Check sheet for the modelled part. Datum: model origin and axes. Units: mm. Face numbers are marked on the shaded views. Round coordinates to 2 decimals unless told otherwise and drop trailing zeros. Write each loop counter-clockwise with the first axis right and the second up, starting at its lowest first coordinate (ties: lowest second). Pieces come first, ordered by that corner, then holes. Notation, with made-up numbers: (19, 24) -> (65, 24) arc R21 ccw to (65, 44) -> close; hole circle Ø6 at (54.5, -36). An arc over 180 degrees is marked (long way). Answer as a JSON object with one key per item and string values. Group by question number.
```python
from build123d import *

# Parameters (mm, degrees)
BOSS_EXTRUDE1_START  = -59.6
SKETCH1_R            = 9
BOSS_EXTRUDE1_DEPTH  = 4
BOSS_EXTRUDE2_START  = -58
SKETCH2_W            = 4
SKETCH2_H            = 49
BOSS_EXTRUDE2_DEPTH  = 12
BOSS_EXTRUDE3_START  = -76.9
SKETCH3_W            = 4
SKETCH3_H            = 22
BOSS_EXTRUDE3_DEPTH  = 39
BOSS_EXTRUDE4_START  = -57.4
SKETCH4_R            = 4.6
BOSS_EXTRUDE4_DEPTH  = 2.3
BOSS_EXTRUDE5_START  = -55.3
SKETCH5_W            = 2.3
SKETCH5_H            = 17.5
BOSS_EXTRUDE5_DEPTH  = 6.6
BOSS_EXTRUDE6_START  = -52.9
SKETCH6_W            = 6
SKETCH6_H            = 10.5
BOSS_EXTRUDE6_DEPTH  = 1.8
BOSS_EXTRUDE7_START  = -55.3
SKETCH7_W            = 2.3
SKETCH7_H            = 17.5
BOSS_EXTRUDE7_DEPTH  = 6.6
BOSS_EXTRUDE8_START  = -52.9
SKETCH8_W            = 6
SKETCH8_H            = 10.5
BOSS_EXTRUDE8_DEPTH  = 1.8
BOSS_EXTRUDE9_START  = -60.6
SKETCH9_R            = 3
BOSS_EXTRUDE9_DEPTH  = 6
BOSS_EXTRUDE10_START = -69.1
SKETCH10_W           = 6
SKETCH10_H           = 13
BOSS_EXTRUDE10_DEPTH = 23.4
BOSS_EXTRUDE11_START = -72.925
SKETCH11_W           = 6
SKETCH11_H           = 2
BOSS_EXTRUDE11_DEPTH = 2.9
BOSS_EXTRUDE12_START = -44.775
SKETCH12_W           = 6
SKETCH12_H           = 2
BOSS_EXTRUDE12_DEPTH = 2.9


with BuildPart() as part:
    # Sketch1 → Boss-Extrude1 (new body)
    with BuildSketch(Plane(origin=(0, 0, 0), x_dir=(0, 0, -1), z_dir=(1, 0, 0)).offset(BOSS_EXTRUDE1_START)):
        with Locations((52, 18)):
            Circle(SKETCH1_R)
    extrude(amount=BOSS_EXTRUDE1_DEPTH)

    # Sketch2 → Boss-Extrude2 (add)
    with BuildSketch(Plane.XY.offset(BOSS_EXTRUDE2_START)):
        with Locations((-57.6, 12.5)):
            Rectangle(SKETCH2_W, SKETCH2_H)
    extrude(amount=BOSS_EXTRUDE2_DEPTH)

    # Sketch3 → Boss-Extrude3 (add)
    with BuildSketch(Plane.XY.offset(BOSS_EXTRUDE3_START)):
        with Locations((-57.6, -20)):
            Rectangle(SKETCH3_W, SKETCH3_H)
    extrude(amount=BOSS_EXTRUDE3_DEPTH)


with BuildPart() as body_2:
    # Sketch4 → Boss-Extrude4 (new body)
    with BuildSketch(Plane(origin=(0, 0, 0), x_dir=(0, 0, -1), z_dir=(1, 0, 0)).offset(BOSS_EXTRUDE4_START)):
        with Locations((52, 18)):
            Circle(SKETCH4_R)
    extrude(amount=BOSS_EXTRUDE4_DEPTH)


with BuildPart() as part_1:
    add(part.part)

    # Combine1: cut body 2
    add(body_2.part, mode=Mode.SUBTRACT)


with BuildPart() as body_2_2:
    # Sketch5 → Boss-Extrude5 (new body)
    with BuildSketch(Plane.XY.offset(BOSS_EXTRUDE5_START)):
        with Locations((-56.25, 26.75)):
            Rectangle(SKETCH5_W, SKETCH5_H)
    extrude(amount=BOSS_EXTRUDE5_DEPTH)


with BuildPart() as part_2:
    add(part_1.part)

    # Combine2: cut body 2 2
    add(body_2_2.part, mode=Mode.SUBTRACT)


with BuildPart() as body_2_3:
    # Sketch6 → Boss-Extrude6 (new body)
    with BuildSketch(Plane.XY.offset(BOSS_EXTRUDE6_START)):
        with Locations((-57.6, 28.75)):
            Rectangle(SKETCH6_W, SKETCH6_H)
    extrude(amount=BOSS_EXTRUDE6_DEPTH)


with BuildPart() as part_3:
    add(part_2.part)

    # Combine3: cut body 2 3
    add(body_2_3.part, mode=Mode.SUBTRACT)


with BuildPart() as body_2_4:
    # Sketch7 → Boss-Extrude7 (new body)
    with BuildSketch(Plane.XY.offset(BOSS_EXTRUDE7_START)):
        with Locations((-56.25, 9.25)):
            Rectangle(SKETCH7_W, SKETCH7_H)
    extrude(amount=BOSS_EXTRUDE7_DEPTH)


with BuildPart() as part_4:
    add(part_3.part)

    # Combine4: cut body 2 4
    add(body_2_4.part, mode=Mode.SUBTRACT)


with BuildPart() as body_2_5:
    # Sketch8 → Boss-Extrude8 (new body)
    with BuildSketch(Plane.XY.offset(BOSS_EXTRUDE8_START)):
        with Locations((-57.6, 7.25)):
            Rectangle(SKETCH8_W, SKETCH8_H)
    extrude(amount=BOSS_EXTRUDE8_DEPTH)


with BuildPart() as part_5:
    add(part_4.part)

    # Combine5: cut body 2 5
    add(body_2_5.part, mode=Mode.SUBTRACT)


with BuildPart() as body_2_6:
    # Sketch9 → Boss-Extrude9 (new body)
    with BuildSketch(Plane(origin=(0, 0, 0), x_dir=(0, 0, -1), z_dir=(1, 0, 0)).offset(BOSS_EXTRUDE9_START)):
        with Locations((52, 18)):
            Circle(SKETCH9_R)
    extrude(amount=BOSS_EXTRUDE9_DEPTH)


with BuildPart() as part_6:
    add(part_5.part)

    # Combine6: cut body 2 6
    add(body_2_6.part, mode=Mode.SUBTRACT)


with BuildPart() as body_2_7:
    # Sketch10 → Boss-Extrude10 (new body)
    with BuildSketch(Plane.XY.offset(BOSS_EXTRUDE10_START)):
        with Locations((-57.6, -20)):
            Rectangle(SKETCH10_W, SKETCH10_H)
    extrude(amount=BOSS_EXTRUDE10_DEPTH)


with BuildPart() as part_7:
    add(part_6.part)

    # Combine7: cut body 2 7
    add(body_2_7.part, mode=Mode.SUBTRACT)


with BuildPart() as body_2_8:
    # Sketch11 → Boss-Extrude11 (new body)
    with BuildSketch(Plane.XY.offset(BOSS_EXTRUDE11_START)):
        with Locations((-57.6, -20)):
            Rectangle(SKETCH11_W, SKETCH11_H)
    extrude(amount=BOSS_EXTRUDE11_DEPTH)


with BuildPart() as part_8:
    add(part_7.part)

    # Combine8: cut body 2 8
    add(body_2_8.part, mode=Mode.SUBTRACT)


with BuildPart() as body_2_9:
    # Sketch12 → Boss-Extrude12 (new body)
    with BuildSketch(Plane.XY.offset(BOSS_EXTRUDE12_START)):
        with Locations((-57.6, -20)):
            Rectangle(SKETCH12_W, SKETCH12_H)
    extrude(amount=BOSS_EXTRUDE12_DEPTH)


with BuildPart() as part_9:
    add(part_8.part)

    # Combine9: cut body 2 9
    add(body_2_9.part, mode=Mode.SUBTRACT)


solid = part_9.part
```
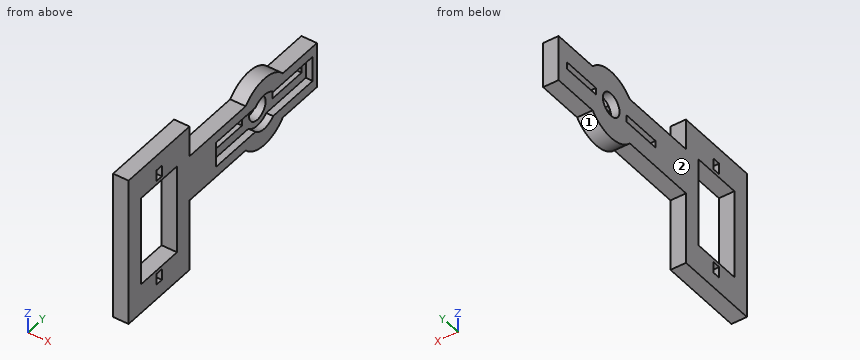
(1) Release check for a two-part mould opening along Y. For the marked faces 1 and 2 record: pulls with the +Y half, pulls with the -Y half, needs draft (parallel to the pull), parting line crosses it, or undercut.
(2) Section check A-A on x = -56.5. State how many separate pieces and enclosed holes the cut face has, then the cut area to 3 significant figures.
(3) Section check C-C on y = 8.5. Record the cut outline in (x, z), then the cut area to 3 significant figures.
(4) Scan lines: line 1 along Y through (x, z) = (-58.6, -52); line 2 along Z through (x, y) = (-57.7, 9.5); line 3 along Y through (x, z) = (-58.2, -68). Record each from-to range of solid material in increasing order.
(5) Section check B-B on z = -52. Record the cut outline in (x, y).
(6) Section check D-D on y = 18. Record the cut outline in (x, z).
(7) Go/stop test with flat-tipped pins: pin 1 Ø0.9 at (x, y) = (-56.5, 28.5) entering from -Z; pin 2 Ø0.9 at (x, y) = (-56.5, 4.5) entering from +Z; pin 3 Ø1.5 at (x, z) = (-56.5, -71.5) entering from +Y. Record where each tip stops, or that it passes through.
Data:
{
 "1": {"face 1": "undercut", "face 2": "needs draft"},
 "2": {"separate pieces": "1", "enclosed holes": "4", "area": "907 mm²"},
 "3": {"outline": "(-59.6, -58) -> (-55.6, -58) -> (-55.6, -55.3) -> (-57.4, -55.3) -> (-57.4, -52.9) -> (-59.6, -52.9) -> close; (-59.6, -51.1) -> (-57.4, -51.1) -> (-57.4, -48.7) -> (-55.6, -48.7) -> (-55.6, -46) -> (-59.6, -46) -> close", "area": "32.2 mm²"},
 "4": {"line 1": "y = -31 to -26.5, -13.5 to 2, 12.5 to 15, 21 to 23.5, 34 to 37", "line 2": "z = -58 to -52.9, -51.1 to -46", "line 3": "y = -31 to -26.5, -13.5 to -9"},
 "5": {"outline": "(-59.6, -31) -> (-55.6, -31) -> (-55.6, -26.5) -> (-59.6, -26.5) -> close; (-59.6, -13.5) -> (-55.6, -13.5) -> (-55.6, 0.5) -> (-57.4, 0.5) -> (-57.4, 2) -> (-59.6, 2) -> close; (-59.6, 12.5) -> (-57.4, 12.5) -> (-57.4, 15) -> (-59.6, 15) -> close; (-59.6, 21) -> (-57.4, 21) -> (-57.4, 23.5) -> (-59.6, 23.5) -> close; (-59.6, 34) -> (-57.4, 34) -> (-57.4, 35.5) -> (-55.6, 35.5) -> (-55.6, 37) -> (-59.6, 37) -> close"},
 "6": {"outline": "(-59.6, -61) -> (-55.6, -61) -> (-55.6, -56.6) -> (-57.4, -56.6) -> (-57.4, -55) -> (-59.6, -55) -> close; (-59.6, -49) -> (-57.4, -49) -> (-57.4, -47.4) -> (-55.6, -47.4) -> (-55.6, -43) -> (-59.6, -43) -> close"},
 "7": {"pin 1": "stops at z = -58", "pin 2": "stops at z = -46", "pin 3": "stops at y = -9"}
}
